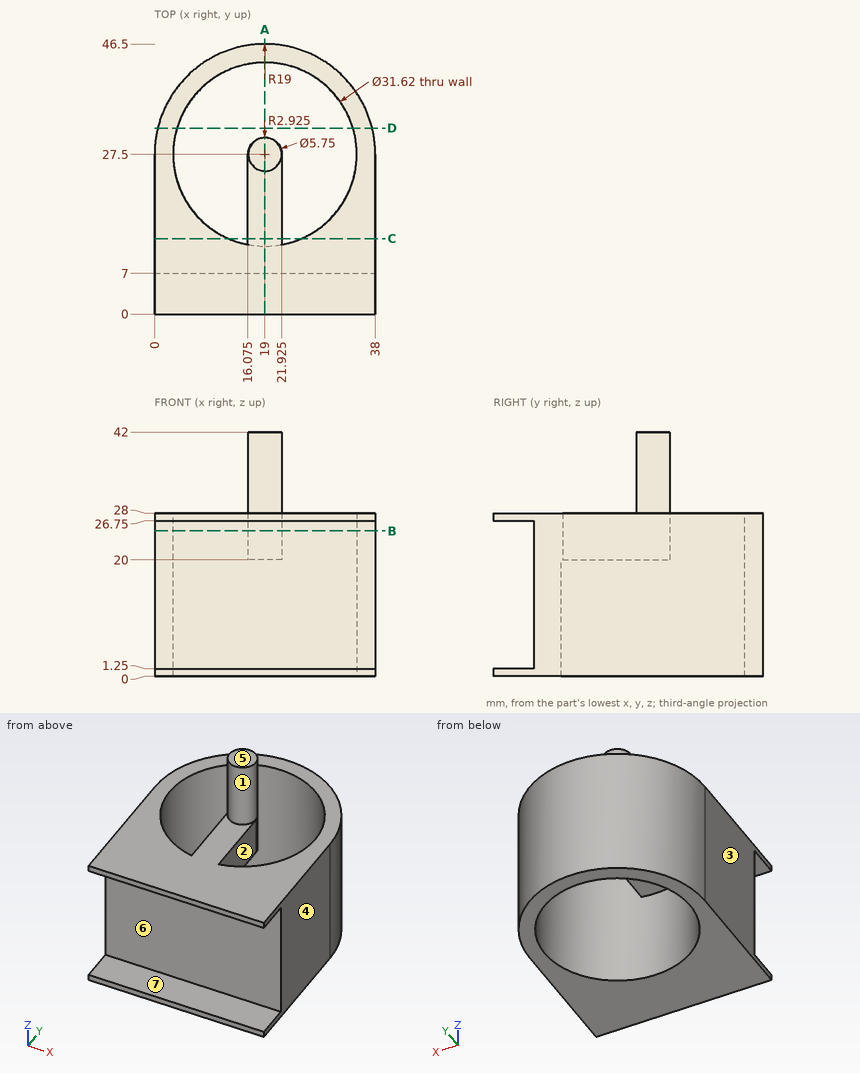
Design review of the part shown in the three views and the two pictorial views. Dimensions are in mm from the part's minimum x, y and z. A direction names the side the tool comes from. Round coordinates to 2 decimals unless told otherwise and drop trailing zeros. Loops run counter-clockwise (first coordinate to the right, second up) from the corner with the lowest first, then second, coordinate; pieces in that order, holes last.
(1) We need section D-D (y = 32). Give the boundary of the cut face in (x, z), plus the area to 3 significant figures.
Returned:
outline: (0.54, 0) - (3.84, 0) - (3.84, 28) - (0.54, 28) - close; (34.16, 0) - (37.46, 0) - (37.46, 28) - (34.16, 28) - close
area: 185 mm2
(2) We need section C-C (y = 13). Give the boundary of the cut face in (x, z) (3 decimals).
Returned:
outline: (0, 0) - (12.699, 0) - (12.699, 28) - (0, 28) - close; (16.075, 20) - (21.925, 20) - (21.925, 28) - (16.075, 28) - close; (25.301, 0) - (38, 0) - (38, 28) - (25.301, 28) - close
(3) We need section B-B (z = 25). Give the boundary of the cut face in (x, y) (3 decimals), plus the area to 3 significant figures.
Returned:
outline: (0, 7) - (38, 7) - (38, 27.5) arc R19 ccw to (0, 27.5) - close; hole (16.075, 11.963) - (16.075, 27.5) arc R2.925 cw to (21.925, 27.5) - (21.925, 11.963) arc R15.81 ccw (long way) to start
area: 666 mm2
(4) Clearance check with flat-ended pins moving along their axes: P1, Ø4, axis at y = 31, z = 22, coming from the +X side; P2, Ø8, axis at x = 13, z = 36.5, coming from the -Y side; P3, Ø4, axis at x = 23.5, y = 22, coming from the -Z side. State where each tip first meets the part, or that it passes through.
Returned:
P1: stops at x = 37.94
P2: stops at y = 25.43
P3: stops at z = 20
(5) Wall thickness on line 1 along X through (y, z) = (27.5, 20.25) (3 decimals); line 2 along Z through (x, y) = (25.5, 3); line 3 along X through (y, z) = (27, 14): over which ranges is each line inside the solid? List them lowest first.
Returned:
line 1: x = 0 to 3.19, 16.075 to 21.925, 34.81 to 38
line 2: z = 0 to 1.25, 26.75 to 28
line 3: x = 0 to 3.2, 34.8 to 38
(6) We need section A-A (x = 19). Give the boundary of the cut face in (y, z) (3 decimals), plus the area to 3 significant figures.
Returned:
outline: (0, 0) - (11.69, 0) - (11.69, 20) - (30.425, 20) - (30.425, 28) - (30.375, 28) - (30.375, 42) - (24.625, 42) - (24.625, 28) - (0, 28) - (0, 26.75) - (7, 26.75) - (7, 1.25) - (0, 1.25) - close; (43.31, 0) - (46.5, 0) - (46.5, 28) - (43.31, 28) - close
area: 469 mm2
(7) Tool access review of the marked faces 1, 2 and 3: name each direction out of +Z, -Z, +X, -X, +Y, -Y from which nothing blocks a thin tool from reaching the whole face with its end or side.
Returned:
face 1: +Z
face 2: +Z, -Z
face 3: +Z, -Z, -X, +Y, -Y
(8) Mouldability with a two-part tool opening along Z and no side actions: class the marked faces 4, 5, 6 and 7 as released by +Z, released by -Z, zero draft, split by the parting line, or undercut.
Returned:
face 4: zero draft
face 5: released by +Z
face 6: undercut
face 7: undercut
